Job drawing, mm, ordinate dimensions from the low corner. One solid piece. A direction names the side the tool comes from. Give positions to 0.01 mm unless a question says otherwise; leave off trailing zeros. Write each loop counter-clockwise with the first axis right and the second up, starting at its lowest first coordinate (ties: lowest second). Pieces come first, ordered by that corner, then holes. Notation, with made-up numbers: (32.25, -22.5) - (38.25, -22.5) arc R32 ccw to (38.25, 11.5) - close; hole circle Ø11 at (52.25, 48). An arc over 180 degrees is marked (long way). Put each result on its own line as item: value. Start each with the question number.
1. Cut at B-B on z = 6.25. List the corners of the cut face in (x, y), and give its area (3 significant figures).
2. Drop flat-ended pins along their axis: pin 1 (1.5 mm diameter, centred on y = 10.5, z = 6.5, fed in from -X); pin 2 (8 mm diameter, centred on x = 15.5, y = 7, fed in from +Z). Give the stop position or say it passes through.
3. Cut at D-D on x = 29.5. List the corners of the cut face in (y, z).
4. Wall check: line 1 (Z direction, x = 29.5, y = 13); line 2 (X direction, y = 11.5, z = 3.75); line 3 (X direction, y = 15, z = 7). Give the ranges that are in metal, low to high.
5. Tool access for the marked faces 3 and 4: list every direction of +Z, -Z, +X, -X, +Y, -Y with a clear straight run to the whole face (end or side of a thin tool).
6. Cut at C-C on x = 37.85. List the corners of the cut face in (y, z).
7. Cut at A-A on y = 10.65. List the corners of the cut face in (x, z).
8. Mould opens along X. For the marked faces 1 and 2 say: +X half, -X half, draft (parallel to the pull), parting line (faces both ways), or undercut.
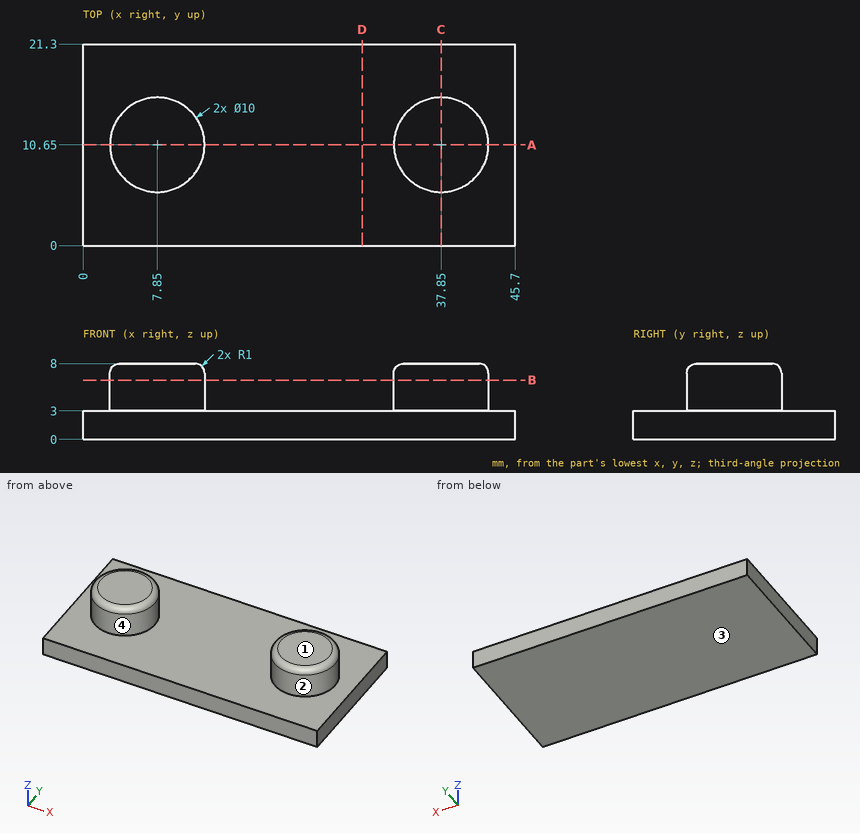
Report:
1. outline: circle Ø10 at (7.85, 10.65); circle Ø10 at (37.85, 10.65)
1. area: 157 mm²
2. pin 1: stops at x = 2.85
2. pin 2: stops at z = 7.88
3. outline: (0, 0) - (21.3, 0) - (21.3, 3) - (0, 3) - close
4. line 1: z = 0 to 3
4. line 2: x = 2.92 to 12.78, 32.92 to 42.78
4. line 3: x = 5.38 to 10.32, 35.38 to 40.32
5. face 3: -Z, +X, -X, +Y, -Y
5. face 4: +Z
6. outline: (0, 0) - (21.3, 0) - (21.3, 3) - (15.65, 3) - (15.65, 7) arc R1 ccw to (14.65, 8) - (6.65, 8) arc R1 ccw to (5.65, 7) - (5.65, 3) - (0, 3) - close
7. outline: (0, 0) - (45.7, 0) - (45.7, 3) - (42.85, 3) - (42.85, 7) arc R1 ccw to (41.85, 8) - (33.85, 8) arc R1 ccw to (32.85, 7) - (32.85, 3) - (12.85, 3) - (12.85, 7) arc R1 ccw to (11.85, 8) - (3.85, 8) arc R1 ccw to (2.85, 7) - (2.85, 3) - (0, 3) - close
8. face 1: draft
8. face 2: undercut
